```python
from build123d import *

# Parameters (mm, degrees)
REDONDEO3_R             = 5
CROQUIS2_R              = 12.5
SALIENTE_EXTRUIR1_DEPTH = 40
CROQUIS3_R              = 20
SALIENTE_EXTRUIR2_DEPTH = 10


with BuildPart() as part:
    # Croquis1 → Revoluci_n1 (revolve)
    with BuildSketch(Plane(origin=(0, 0, 0), x_dir=(1, 0, 0), z_dir=(0, 1, 0)), mode=Mode.PRIVATE) as revoluci_n1_sk:
        with BuildLine():
            Line((93.136469217, 140.438586249), (70, 140.438586249))
            Line((70, 140.438586249), (48.737618848, 131.388343039))
            Line((48.737618848, 131.388343039), (48.737618848, 120.610275725))
            Line((48.737618848, 120.610275725), (31.868809424, 113.430137863))
            Line((31.868809424, 113.430137863), (31.868809424, 102.180137863))
            Line((31.868809424, 102.180137863), (15, 95))
            Line((15, 95), (15, 0))
            Line((15, 0), (70, 0))
            Line((70, 0), (145, 0))
            Line((145, 0), (145, 88.080438356))
            ThreePointArc((145, 88.080438356), (144.820704123, 89.965583051), (144.289245896, 91.783128012))
            Line((144.289245896, 91.783128012), (136.332769552, 111.744202824))
            ThreePointArc((136.332769552, 111.744202824), (135.522244312, 113.34352185), (134.43914749, 114.772393358))
            Line((134.43914749, 114.772393358), (121.382088175, 129.118971571))
            ThreePointArc((121.382088175, 129.118971571), (119.636600305, 130.638907317), (117.588438461, 131.716852417))
            Line((117.588438461, 131.716852417), (96.738443336, 139.767347284))
            ThreePointArc((96.738443336, 139.767347284), (94.968461254, 140.269344367), (93.136469217, 140.438586249))
        make_face()
    revolve(revoluci_n1_sk.sketch.rotate(Axis((-209.218950064, 0, 0), (1, 0, 0)), 180), axis=Axis((-209.218950064, 0, 0), (1, 0, 0)))

    # Redondeo3
    redondeo3_edges = [part.edges().sort_by_distance(p)[0] for p in [
        (15, 0, -95),
        (31.868809424, 0, -102.180137863),
        (31.868809424, 0, -113.430137863),
        (48.737618848, 0, -120.610275725),
        (48.737618848, 0, -131.388343039),
    ]]
    fillet(redondeo3_edges, radius=REDONDEO3_R)

    # Croquis2 → Saliente-Extruir1 (add)
    with BuildSketch(Plane(origin=(145, 0, 0), x_dir=(0, 0, -1), z_dir=(1, 0, 0))):
        Circle(CROQUIS2_R)
    extrude(amount=SALIENTE_EXTRUIR1_DEPTH)

    # Croquis3 → Saliente-Extruir2 (add)
    with BuildSketch(Plane(origin=(185, 0, 0), x_dir=(0, 0, -1), z_dir=(1, 0, 0))):
        Circle(CROQUIS3_R)
    extrude(amount=SALIENTE_EXTRUIR2_DEPTH)


solid = part.part
```
Here's how the part is built. I have some questions about the finished solid (model axes, mm). A direction names the side the tool comes from. Coordinates: 2 decimals unless noted, no trailing zeros. Loops run counter-clockwise (first coordinate to the right, second up) from the corner with the lowest first, then second, coordinate; pieces in that order, holes last. Notation, with made-up numbers: M 78.5,25 L 117.5,25 A7 cw 117.5,38 Z; hole C 7,-0.5 d7. An arc over 180 degrees is marked long. One line per item, written item: value.
1. Will these pins go through, and if not, where does the flat tip stop? pin 1 Ø2 at (x, z) = (125, -6) entering from +Y; pin 2 Ø1.5 at (x, y) = (117, -5.5) entering from +Z; pin 3 Ø2 at (x, y) = (66.5, -52.5) entering from +Z.
Geometry says:
pin 1: stops at y = 126.1
pin 2: stops at z = 132.12
pin 3: stops at z = 129.26
2. Please list where these lines run through material, in increasing order: probe 1 along X at (y, z) = (16, 4.5); probe 2 along X at (y, z) = (44, 47); probe 3 along Z at (x, y) = (99, 44).
Geometry says:
probe 1: x = 15 to 145, 185 to 195
probe 2: x = 15 to 145
probe 3: z = -131.74 to 131.74
3. Imagine slicing it at A-A (x = 105). List the corners of the cut face in (y, z) for me.
Geometry says:
outline: C 0,0 d273.15
4. On a 3-axis mill with a long thin cutter (end or side, diameter ignored), from which of +Z, -Z, +X, -X, +Y, -Y can I reach the whole of each face in a straight line? I mean faces 5 (the flat face through (195, 0, 0)), 6 (the flat face through (48.738, -105, -67)), 7 (the cylindrical face through (189.93, -19.524, 4.336)). Say none if no direction works.
Geometry says:
face 5: +Z, -Z, +X, +Y, -Y
face 6: -X
face 7: +X
5. Thinking about a two-plate mould opening in X: for faces 1 (the flat face through (185, 9, -9)), 2 (the cylindrical face through (164.72, 3.755, -11.923)), 3 (the conical face through (52.66, -5.85, -132.93)), 4 (the cylindrical face through (81.406, -42.184, 133.953)), which applies, +X half, -X half, draft (parallel to the pull), parting line (faces both ways), or undercut?
Geometry says:
face 1: undercut
face 2: undercut
face 3: -X half
face 4: draft
